from build123d import *

# Parameters (mm, degrees)
F1_DEPTH = 25.4
F4_W     = 55.0225842744
F4_H     = 55.1656335513
F5_DEPTH = 50.8


with BuildPart() as f1:
    # F0 (on Front) → F1 (new body)
    with BuildSketch(Plane.XZ):
        Polygon((-68.4096906334, 54.0788695137), (-68.4096906334, -55.1656335513), (80.5874373764, -55.1656335513), (80.5874373764, -31.6427350123), (-44.8120329529, 54.0788695137), align=None)
    extrude(amount=F1_DEPTH)


with BuildPart() as f3_1:
    # F3: instance of F1
    add(f1.part.mirror(Plane.XZ.offset(-25.4)))


with BuildPart() as f1_1:
    add(f1.part)

    add(f3_1.part)  # F5 merges F3_1
    # F4 (on face) → F5 (join, through all)
    with BuildSketch(Plane(origin=(0, 0, 0), x_dir=(-1, 0, 0), z_dir=(0, 1, 0))):
        with Locations((40.8983984962, -27.5828167757)):
            Rectangle(F4_W, F4_H)
    extrude(amount=F5_DEPTH)


solid = f1_1.part
Read the model definition and answer for the solid it produces. Units are mm, in the model's axes. A direction names the side the tool comes from. Coordinates: 2 decimals unless noted, no trailing zeros. Order: outer loops, then holes, each group sorted by start corner. A loop starts at its lowest first (then second) coordinate and runs counter-clockwise, first axis right, second up. Notation, with made-up numbers: M 55.25,3 L 85.25,3 A23 cw 85.25,25 Z; hole C -29,45 d10. An arc over 180 degrees is marked long. Put each result on its own line as item: value. Start each with the question number.
Item 1: Consider probe 1 along Y at (x, z) = (30, -34); probe 2 along X at (y, z) = (7.5, -10); probe 3 along Z at (x, y) = (-35, 7.5). Determine where each line is inside the solid, lowest interval first. Write a range as [from, to].
Item 2: The mould has two halves that part along Y. Classify faces 4 (the face through (-12, 76.2, -12)), 5 (the face through (80.587, -13, -44)), 6 (the face through (5, 50.8, -12)): +Y half, -Y half, draft (parallel to the pull), parting line (faces both ways), or undercut.
Item 3: Section D-D, the plane x = -57 is taken. Determine the outline of the cut face in (y, z).
Item 4: Section A-A, the plane x = 57 is taken. Determine the outline of the cut face in (y, z).
Item 5: Section C-C, the plane y = 66.5 is taken. Determine the outline of the cut face in (x, z).
Item 6: Section B-B, the plane z = 25 is taken. Determine the outline of the cut face in (x, y), plus the area to 3 significant figures.
Item 7: For faces 1 (the face through (-13.387, 25, -28)), 2 (the face through (-41, 25, 0)), 3 (the face through (5, 0, -12)), determine the directions among +Z, -Z, +X, -X, +Y, -Y from which every point of the face is accessible in a straight line to the end or side of a thin tool.
Item 8: Given pin 1 Ø1 at (x, y) = (-2.5, 65) entering from +Z; pin 2 Ø5 at (x, y) = (-27.5, 51.5) entering from +Z; pin 3 Ø1 at (y, z) = (31.5, -18.5) entering from +X, each flat-ended and moving along its own axis, determine where each tip first touches the part or whether it passes through.
Computed:
1. probe 1: y = [-25.4, 0], [50.8, 76.2]
1. probe 2: x = [-68.41, -13.39]
1. probe 3: z = [-55.17, 0]
2. face 4: +Y half
2. face 5: draft
2. face 6: undercut
3. outline: M -25.4,-55.17 L 76.2,-55.17 L 76.2,54.08 L 50.8,54.08 L 50.8,0 L 0,0 L 0,54.08 L -25.4,54.08 Z
4. outline: M -25.4,-55.17 L 0,-55.17 L 0,-15.52 L -25.4,-15.52 Z; M 50.8,-55.17 L 76.2,-55.17 L 76.2,-15.52 L 50.8,-15.52 Z
5. outline: M -68.41,-55.17 L 80.59,-55.17 L 80.59,-31.64 L -44.81,54.08 L -68.41,54.08 Z
6. outline: M -68.41,-25.4 L -2.27,-25.4 L -2.27,0 L -68.41,0 Z; M -68.41,50.8 L -2.27,50.8 L -2.27,76.2 L -68.41,76.2 Z
6. area: 3,360 mm2
7. face 1: +Z, -Z, +X
7. face 2: +Z, +X, -X
7. face 3: +Z, +X
8. pin 1: stops at z = 25.5
8. pin 2: stops at z = 43.95
8. pin 3: stops at x = -13.39
